Autodesk Inventor part; units mm, degrees
ref_plane "YZ Plane" through (0, 0, 0) normal (1, 0, 0) x (0, 1, 0)
ref_plane "XZ Plane" through (0, 0, 0) normal (0, 1, 0) x (-1, 0, 0)
ref_plane "XY Plane" through (0, 0, 0) normal (0, 0, 1) x (1, 0, 0)
sketch "Sketch1" plane through (0, 0, 0) normal (0, 1, 0) x (-1, 0, 0)
  line L0 (-10, 11) -> (10, 11)
  line L1 (10, 11) -> (10, -11)
  line L2 (10, -11) -> (-10, -11)
  line L3 (-10, -11) -> (-10, 11)
  line L4 (-10, 11) -> (10, -11) construction
  line L5 (10, 11) -> (-10, -11) construction
  point P0 (0, 0)
  dimension "d0" = 20
  dimension "d1" = 22
extrude "Extrusion1" add sketch "Sketch1" against normal blind 2
sketch "Sketch2" plane through (0, 0, 0) normal (0, 1, 0) x (1, 0, 0)
  circle A0 centre (1.2, 0) radius 7.5
  line L0 (-10, 11) -> (10, 11)
  line L1 (10, -11) -> (10, 11)
  dimension "d4" = 15
  dimension "d10" = 8.8
extrude "Extrusion2" add sketch "Sketch2" along normal blind 16
sketch "Sketch3" plane through (0, 0, 0) normal (0, 1, 0) x (1, 0, 0)
  line L0 (-10, -8.4) -> (-10, -11)
  circle A0 centre (-5.4, -8.4) radius 1.6
  circle A1 centre (7.4, 8.4) radius 1.6
  point P0 (0, 0)
  point P1 (10, 11)
  dimension "d9" = 3.2
  dimension "d13" = 3.2
extrude "Extrusion3" cut sketch "Sketch3" against normal up to surface (2 mm away)
properties part number "SONIC"
Here's how the part is built. I have some questions about the finished solid (model axes, mm). A direction names the side the tool comes from. Give positions to 0.01 mm unless a question says otherwise; leave off trailing zeros. Loops run counter-clockwise (first coordinate to the right, second up) from the corner with the lowest first, then second, coordinate; pieces in that order, holes last. Notation, with made-up numbers: (8.5, -35) -> (37.5, -35) arc R16 ccw to (37.5, -30) -> close; hole circle Ø9 at (9.25, -17.5). An arc over 180 degrees is marked (long way). Answer as a JSON object with one key per item and string values. Group by question number.
Item 1: I need wall thicknesses on L1, parallel to X at y = -1.3, z = -8.4; L2, parallel to Z at x = 7.4, y = -0.75; L3, parallel to Z at x = -5.4, y = -1.45. Which ranges of each line are inside material? Lowest first, please.
Item 2: Imagine slicing it at C-C on z = 0. Write out the boundary of the cut face in (x, y), then the cut area to 3 significant figures.
Item 3: Imagine slicing it at D-D on y = -0.5. Write out the boundary of the cut face in (x, z).
Item 4: Imagine slicing it at A-A on z = -8.4. Write out the boundary of the cut face in (x, y).
Item 5: On a 3-axis mill with a long thin cutter (end or side, diameter ignored), from which of +Z, -Z, +X, -X, +Y, -Y can I reach the whole of each face in a straight line? I mean faces 5 (the flat face through (-7, 0, 0)), 6 (the flat face through (0, -1, 11)). Say none if no direction works.
Item 6: Will these pins go through, and if not, where does the flat tip stop? pin 1 (1.5 mm diameter, centred on x = 4.5, y = 2.5, fed in from -Z); pin 2 (10 mm diameter, centred on x = 4, y = 5.5, fed in from +Z); pin 3 (1 mm diameter, centred on x = -3, y = 9, fed in from -Z).
Item 7: Thinking about a two-plate mould opening in Z: for faces 1 (the cylindrical face through (8.354, 7.888, 2.253)), 2 (the flat face through (0, -1, -11)), 3 (the cylindrical face through (-5.608, -0.986, 6.814)), 4 (the flat face through (1, 16, 0)), which applies, pulls with the +Z half, pulls with the -Z half, needs draft (parallel to the pull), parting line crosses it, or undercut?
Item 8: Imagine slicing it at B-B on x = -5.4. Write out the boundary of the cut face in (y, z), then the cut area to 3 significant figures.
Answer list:
{
 "1": {"L1": "x = -10 to 5.8, 9 to 10", "L2": "z = -11 to -10, -6.8 to 11", "L3": "z = -11 to 6.8, 10 to 11"},
 "2": {"outline": "(-10, -2) -> (10, -2) -> (10, 0) -> (8.7, 0) -> (8.7, 16) -> (-6.3, 16) -> (-6.3, 0) -> (-10, 0) -> close", "area": "280 mm2"},
 "3": {"outline": "(-10, -11) -> (10, -11) -> (10, 11) -> (-10, 11) -> close; hole circle Ø3.2 at (-5.4, 8.4); hole circle Ø3.2 at (7.4, -8.4)"},
 "4": {"outline": "(-10, -2) -> (5.8, -2) -> (5.8, 0) -> (-10, 0) -> close; (9, -2) -> (10, -2) -> (10, 0) -> (9, 0) -> close"},
 "5": {"face 5": "+Y", "face 6": "+Z, +X, -X, +Y, -Y"},
 "6": {"pin 1": "stops at z = -7.05", "pin 2": "stops at z = 7.5", "pin 3": "stops at z = -6.52"},
 "7": {"face 1": "parting line crosses it", "face 2": "pulls with the -Z half", "face 3": "undercut", "face 4": "needs draft"},
 "8": {"outline": "(-2, -11) -> (0, -11) -> (0, -3.56) -> (16, -3.56) -> (16, 3.56) -> (0, 3.56) -> (0, 6.8) -> (-2, 6.8) -> close; (-2, 10) -> (0, 10) -> (0, 11) -> (-2, 11) -> close", "area": "152 mm2"}
}
